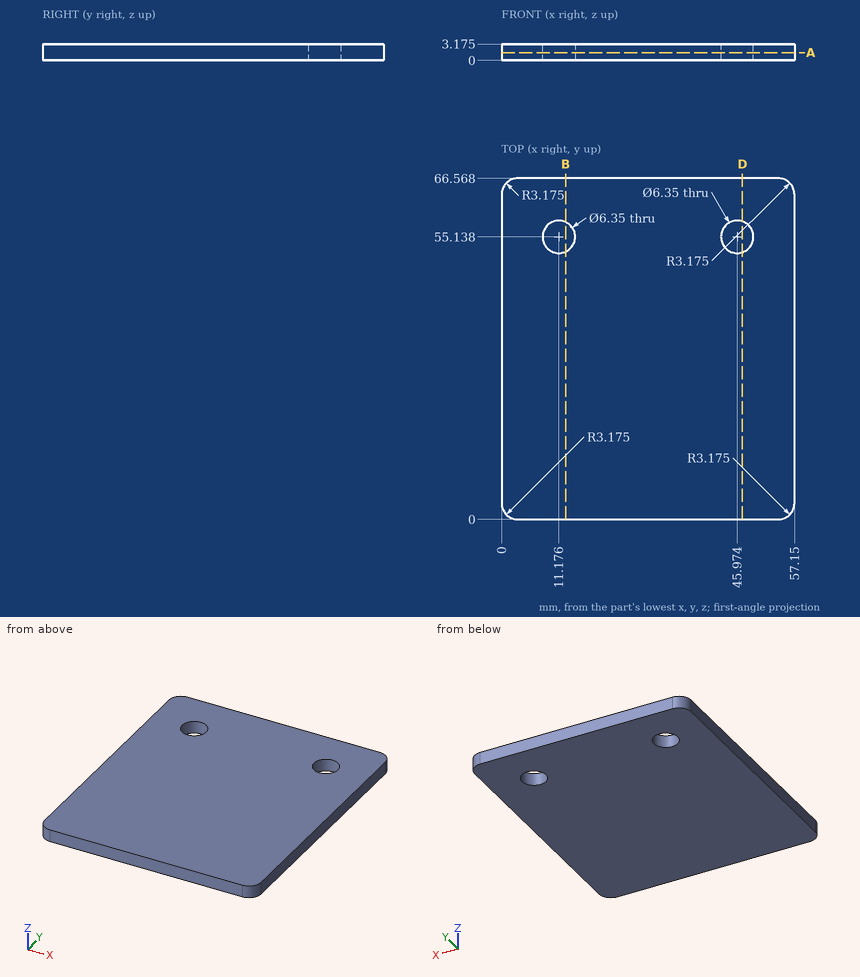
Job drawing, mm, ordinate dimensions from the low corner. One solid piece. Give positions to 0.01 mm unless a question says otherwise; leave off trailing zeros. Order: outer loops, then holes, each group sorted by start corner. A loop starts at its lowest first (then second) coordinate and runs counter-clockwise, first axis right, second up. Notation, with made-up numbers: (-28, 30.25) -> (11, 30.25) arc R17 cw to (11, 58.25) -> close; hole circle Ø6 at (18.25, 37.25). An arc over 180 degrees is marked (long way). Return JSON: item names as keys, results as strings.
Q1. Drill centre lines: line 1 (X direction, y = 55, z = 2.5); line 2 (Y direction, x = 3, z = 2.15) (1 decimal); line 3 (Y direction, x = 47, z = 2.95). Where is each one in solid material? Low to high.
Working result:
{"line 1": "0 to 8, 14.35 to 42.8, 49.15 to 57.15", "line 2": "0 to 66.6", "line 3": "0 to 52.13, 58.14 to 66.57"}
Q2. Saw through at A-A (z = 1.5). Count the separate pieces of the cut face and the enclosed holes in it, then the cut area to 3 significant figures.
Working result:
{"separate pieces": "1", "enclosed holes": "2", "area": "3,730 mm²"}
Q3. Saw through at D-D (x = 47). Write the cut outline in (y, z) (1 decimal).
Working result:
{"outline": "(0, 0) -> (52.1, 0) -> (52.1, 3.2) -> (0, 3.2) -> close; (58.1, 0) -> (66.6, 0) -> (66.6, 3.2) -> (58.1, 3.2) -> close"}
Q4. Saw through at B-B (x = 12.5). Write the cut outline in (y, z) (1 decimal), then the cut area to 3 significant figures.
Working result:
{"outline": "(0, 0) -> (52.3, 0) -> (52.3, 3.2) -> (0, 3.2) -> close; (58, 0) -> (66.6, 0) -> (66.6, 3.2) -> (58, 3.2) -> close", "area": "193 mm²"}
